Source: three-view drawing plus pictorial views. Frame: mm from the lowest corner of the part. A direction names the side the tool comes from. Round coordinates to 2 decimals unless told otherwise and drop trailing zeros. Write each loop counter-clockwise with the first axis right and the second up, starting at its lowest first coordinate (ties: lowest second). Pieces come first, ordered by that corner, then holes. Notation, with made-up numbers: M 5.5,-7.75 L 63.5,-7.75 A18 ccw 63.5,14.25 Z; hole C 62.25,18.5 d4. An arc over 180 degrees is marked long. Put each result on its own line as item: value. Start each with the question number.
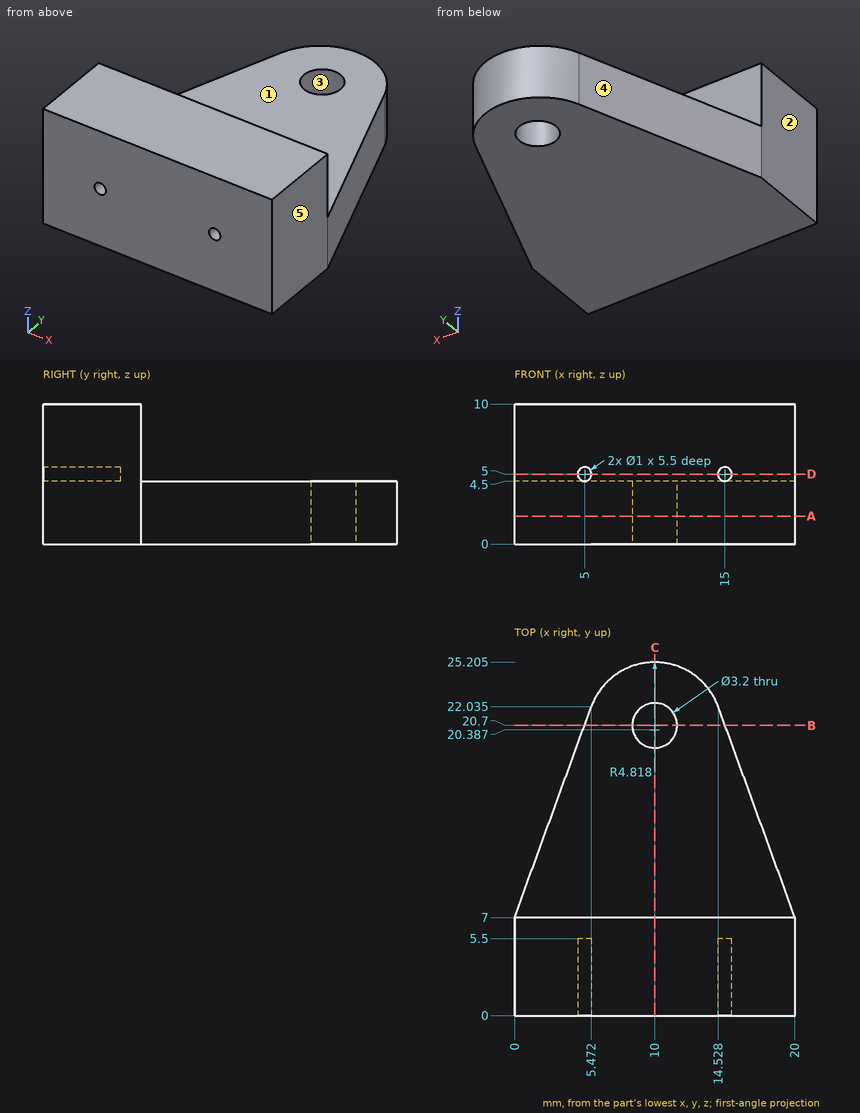
(1) Section query A-A (z = 2). Return loops of the section in (x, y) (1 decimal), and give its area (3 significant figures).
(2) Contact query for flat-ended pins moving along their axis: P1, Ø0.8, axis at x = 15, z = 5, coming from the -Y side; P2, Ø3, axis at x = 4.5, y = 14.5, coming from the +Z side; P3, Ø3, axis at x = 8, z = 7, coming from the +Y side. Output: stop coordinate, or through.
(3) Section query D-D (z = 5). Return loops of the section in (x, y), and give its area (3 significant figures).
(4) Access query for the marked faces 1 and 2. Directions: +Z, -Z, +X, -X, +Y, -Y. A direction counts if a zero-diameter tool reaches every point of the face in a straight line with its end or side. Return the directions, or none.
(5) Section query C-C (x = 10). Return loops of the section in (y, z) (1 decimal).
(6) Ray query, line 1 along Y through (x, z) = (10, 2.9) (1 decimal); line 2 along Z through (x, y) = (15, 2.7); line 3 along Y through (x, z) = (18.5, 8.25). Return the intervals inside material, ascending.
(7) Pull-direction query (X, two-part tool) for the marked faces 3, 4 and 5; classes: +X half, -X half, draft (parallel to the pull), parting line (faces both ways), or undercut.
(8) Section query B-B (y = 20.7). Return loops of the section in (x, z).
Entries:
1. outline: M 0,0 L 20,0 L 20,7 L 14.5,22 A4.8 ccw 5.5,22 L 0,7 Z; hole C 10,20.7 d3.2
1. area: 371 mm2
2. P1: y = 5.5
2. P2: z = 4.5
2. P3: y = 7
3. outline: M 0,0 L 4.5,0 L 4.5,5.5 L 5.5,5.5 L 5.5,0 L 14.5,0 L 14.5,5.5 L 15.5,5.5 L 15.5,0 L 20,0 L 20,7 L 0,7 Z
3. area: 129 mm2
4. face 1: +Z, +X, -X, +Y
4. face 2: +Z, -Z, -X, +Y, -Y
5. outline: M 0,0 L 19.1,0 L 19.1,4.5 L 7,4.5 L 7,10 L 0,10 Z; M 22.3,0 L 25.2,0 L 25.2,4.5 L 22.3,4.5 Z
6. line 1: 0 to 19.1, 22.3 to 25.2
6. line 2: 0 to 4.5, 5.5 to 10
6. line 3: 0 to 7
7. face 3: undercut
7. face 4: -X half
7. face 5: +X half
8. outline: M 4.99,0 L 8.4,0 L 8.4,4.5 L 4.99,4.5 Z; M 11.6,0 L 15.01,0 L 15.01,4.5 L 11.6,4.5 Z
